```python
from build123d import *

# Parameters (mm, degrees)
SKETCH2_W               = 68
SKETCH2_H               = 68
CUT_EXTRUDE1_DEPTH      = 6
CUT_EXTRUDE1_DEPTH_BACK = 6


with BuildPart() as part:
    # Sketch1 → Revolve1 (revolve)
    with BuildSketch(Plane.XY):
        Polygon((0, 0), (8.45, 0), (17.780127019, -2.5), (8.45, -5), (0, -5), align=None)
    revolve(axis=Axis((0, -5, 0), (0, 1, 0)))

    # Sketch2 → Cut-Extrude1 (cut, two sides)
    with BuildSketch(Plane(origin=(0, 0, 0), x_dir=(1, 0, 0), z_dir=(0, 1, 0))) as cut_extrude1_sk:
        Rectangle(SKETCH2_W, SKETCH2_H)
        Polygon((-8.5, -4.907477288), (0, -9.814954576), (8.5, -4.907477288), (8.5, 4.907477288), (0, 9.814954576), (-8.5, 4.907477288), align=None, mode=Mode.SUBTRACT)
    extrude(amount=CUT_EXTRUDE1_DEPTH, mode=Mode.SUBTRACT)
    extrude(cut_extrude1_sk.sketch, amount=-CUT_EXTRUDE1_DEPTH_BACK, mode=Mode.SUBTRACT)

    # Sketch3 → Cut-Revolve1 (revolve, cut)
    with BuildSketch(Plane.XY):
        Polygon((0, 0), (5, 0), (4.3235, -0.6765), (4.3235, -4.3235), (5, -5), (0, -5), align=None)
    revolve(axis=Axis((0, -5, 0), (0, 1, 0)), mode=Mode.SUBTRACT)


solid = part.part
```
Read the model definition and answer for the solid it produces. Units are mm, in the model's axes. Give positions to 0.01 mm unless a question says otherwise; leave off trailing zeros. Order: outer loops, then holes, each group sorted by start corner. A loop starts at its lowest first (then second) coordinate and runs counter-clockwise, first axis right, second up.
(1) Given pin 1 (3 mm diameter, centred on x = 4, y = -1.5, fed in from +Z), flat-ended and moving along its own axis, determine where the tip first touches the part or whether it passes through.
(2) Find section A-A (z = 0). Give the vertices of the cut face in (x, y), plus the area to 3 significant figures.
(3) Find section B-B (y = -2.6). Give the vertices of the cut face in (x, z).
(4) For a pull along X with two mould halves and no side action, classify faces 1 (the cylindrical face through (-3.43, -2.53, 2.63)), 2 (the flat face through (4.191, -2.465, 7.396)), 3 (the flat face through (-8.5, -2, 0)) as released by +X, released by -X, zero draft, split by the parting line, or undercut.
(5) Straight lines are drawn through the part: L1, parallel to X at y = -2.95, z = 0; L2, parallel to Z at x = 3, y = -4.05; L3, parallel to Z at x = 0.5, y = -3.35. For each, find the intervals that lie inside material, in ascending order.
Result sheet:
1. pin 1: stops at z = 8.37
2. outline: (-8.5, -4.99) - (-8.45, -5) - (-5, -5) - (-4.32, -4.32) - (-4.32, -0.68) - (-5, 0) - (-8.45, 0) - (-8.5, -0.01) - close; (4.32, -4.32) - (5, -5) - (8.45, -5) - (8.5, -4.99) - (8.5, -0.01) - (8.45, 0) - (5, 0) - (4.32, -0.68) - close
2. area: 40.8 mm2
3. outline: (-8.5, -4.91) - (0, -9.81) - (8.5, -4.91) - (8.5, 4.91) - (0, 9.81) - (-8.5, 4.91) - close; hole circle Ø8.65 at (0, 0)
4. face 1: undercut
4. face 2: released by +X
4. face 3: released by -X
5. L1: x = -8.5 to -4.32, 4.32 to 8.5
5. L2: z = -8.08 to -3.11, 3.11 to 8.08
5. L3: z = -9.53 to -4.29, 4.29 to 9.53
